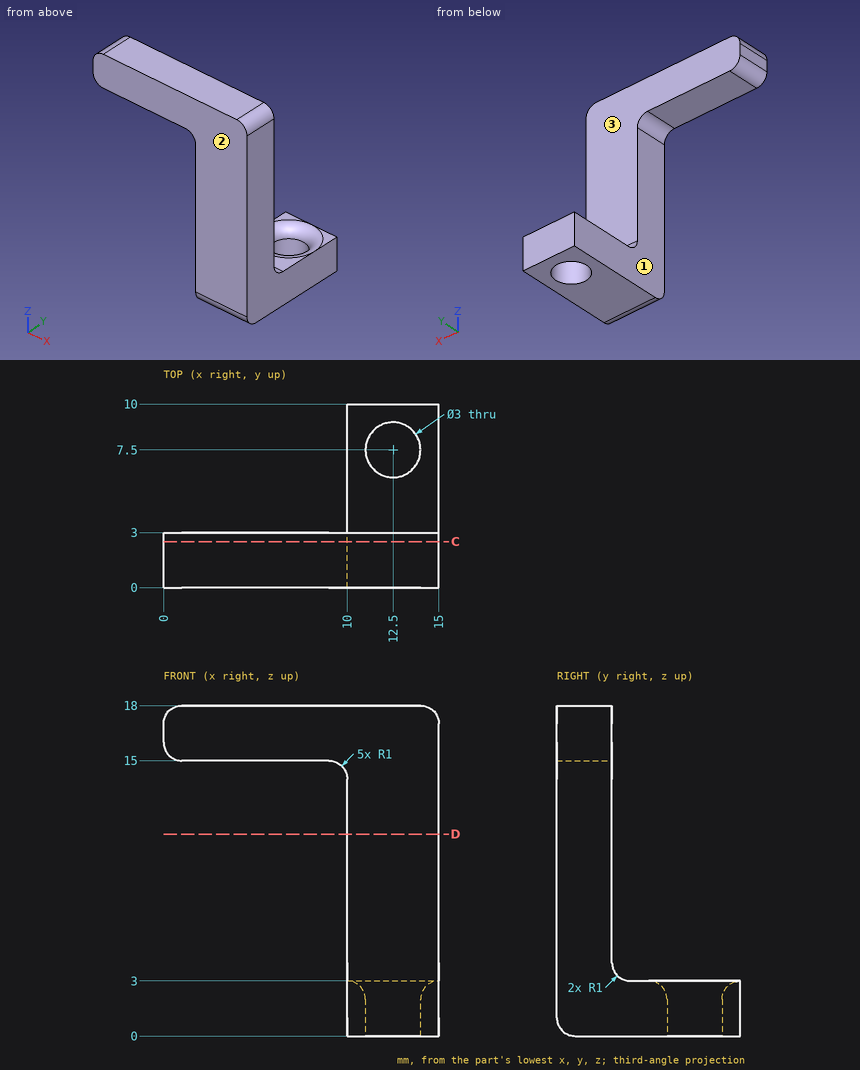
Could you check a few things on this drawing? It's one solid part, dimensions in mm from its lowest x, y, z. A direction names the side the tool comes from. Give positions to 0.01 mm unless a question says otherwise; leave off trailing zeros. Loops run counter-clockwise (first coordinate to the right, second up) from the corner with the lowest first, then second, coordinate; pieces in that order, holes last. Notation, with made-up numbers: (41, -37.5) -> (58, -37.5) arc R30 ccw to (58, -13.5) -> close; hole circle Ø10 at (14.25, -24.5). An arc over 180 degrees is marked (long way). Use one line per item in the form item = value. Start each with the question number.
1) Imagine slicing it at C-C (y = 2.5). Please give me the cut outline in (x, z), then the cut area to 3 significant figures.
2) Which directions (+Z, -Z, +X, -X, +Y, -Y) give clear straight access to the entire face, cutting with the end or side of a thin tool? Please do the marked faces 1, 2 and 3.
3) Please list where these lines run through material, in increasing order: line 1 along Y through (x, z) = (12.5, 15.5); line 2 along Z through (x, y) = (4.25, 2); line 3 along Y through (x, z) = (12.5, 1.35).
4) Imagine slicing it at D-D (z = 11). Please give me the cut outline in (x, y).
5) For P1, Ø4, axis at x = 13.5, y = 6, coming from the +Z side; P2, Ø8, axis at x = 11.5, z = 4.5, coming from the +Y side; P3, Ø1, axis at y = 4, z = 3, coming from the -X side; P4, Ø8, axis at x = 11, z = 7.5, coming from the +Y side, each with a flat end and sliding along its axis, tell me the tip position at first contact or that it passes through.
Check values:
q1.outline = (0, 16) arc R1 ccw to (1, 15) -> (9, 15) arc R1 cw to (10, 14) -> (10, 0) -> (15, 0) -> (15, 17) arc R1 ccw to (14, 18) -> (1, 18) arc R1 ccw to (0, 17) -> close
q1.area = 120 mm^2
q2.face_1 = -Z, -X, +Y, -Y
q2.face_2 = +Z, -Z, +X, -X, -Y
q2.face_3 = +Z, +X, -X, +Y
q3.line_1 = 0 to 3
q3.line_2 = 15 to 18
q3.line_3 = 0 to 6, 9 to 10
q4.outline = (10, 0) -> (15, 0) -> (15, 3) -> (10, 3) -> close
q5.P1 = 3
q5.P2 = 10
q5.P3 = 10
q5.P4 = 3.13
